Input: part model. Units: mm. Frame: model coordinates. Face numbers are marked on the shaded views. A direction names the side the tool comes from. Give positions to 0.01 mm unless a question says otherwise; leave off trailing zeros. Loops run counter-clockwise (first coordinate to the right, second up) from the corner with the lowest first, then second, coordinate; pieces in that order, holes last. Notation, with made-up numbers: (74.5, 19.25) -> (95.5, 19.25) arc R15 cw to (95.5, 32.25) -> close; hole circle Ø1 at (63.25, 64). An arc over 180 degrees is marked (long way). Answer in a Markdown table with one row per item. Add a question column.
```python
from build123d import *

# Parameters (mm, degrees)
BOSS_EXTRUDE1_DEPTH       = 20
SHELL1_T                  = -3.3
SHELL1_THICKNESS_2_FACE_W = 33.4
SHELL1_THICKNESS_2_FACE_H = 36.7
SHELL1_THICKNESS_2_DEPTH  = 6.7
SHELL1_THICKNESS_3_FACE_W = 36.7
SHELL1_THICKNESS_3_FACE_H = 33.4
SHELL1_THICKNESS_3_DEPTH  = 3.1
CUT_EXTRUDE1_REACH        = 84.439
SKETCH2_R                 = 6.65
CUT_EXTRUDE2_REACH        = 74.967
SKETCH3_R                 = 6.65
FILLET1_R                 = 2


with BuildPart() as part:
    # Sketch1 → Boss-Extrude1 (new, symmetric)
    with BuildSketch(Plane.XY):
        Polygon((0, -24), (0, 0), (16.970562748, 16.970562748), (-11.313708499, 45.254833996), (-40, 16.568542495), (-40, -24), align=None)
    extrude(amount=BOSS_EXTRUDE1_DEPTH, both=True)

    # Shell1
    shell1_openings = [part.faces().sort_by_distance(p)[0] for p in [
        (-40, -3.715728753, 0),
        (-25.656854249, 30.911688245, 0),
    ]]
    offset(amount=SHELL1_T, openings=shell1_openings, kind=Kind.INTERSECTION)

    # Shell1 thickness 2 face (on inner face of the shell) → Shell1 thickness 2 (add)
    with BuildSketch(Plane(origin=(-21.65, -20.7, 0), x_dir=(0, 0, -1), z_dir=(0, -1, 0))):
        Rectangle(SHELL1_THICKNESS_2_FACE_W, SHELL1_THICKNESS_2_FACE_H)
    extrude(amount=-SHELL1_THICKNESS_2_DEPTH)

    # Shell1 thickness 3 face (on inner face of the shell) → Shell1 thickness 3 (add)
    with BuildSketch(Plane(origin=(-0.671751442, 29.945972183, 0), x_dir=(-0.707106781187, 0.707106781187, 0), z_dir=(0.707106781187, 0.707106781187, 0))):
        Rectangle(SHELL1_THICKNESS_3_FACE_W, SHELL1_THICKNESS_3_FACE_H)
    extrude(amount=-SHELL1_THICKNESS_3_DEPTH)

    # Sketch2 → Cut-Extrude1 (cut, up to next)
    with BuildSketch(Plane.XZ.offset(24), mode=Mode.PRIVATE) as cut_extrude1_sk1:
        with Locations(Location((-20, 0, 0), (0, 0, 270))):
            Circle(SKETCH2_R)
    cut_extrude1_tool1 = extrude(cut_extrude1_sk1.sketch, amount=-CUT_EXTRUDE1_REACH, mode=Mode.PRIVATE) & part.part
    add(cut_extrude1_tool1.solids().sort_by_distance((-20, -24, 0))[0], mode=Mode.SUBTRACT)

    # Sketch3 → Cut-Extrude2 (cut, up to next)
    with BuildSketch(Plane(origin=(16.970562748, 16.970562748, 0), x_dir=(0, 0, -1), z_dir=(0.7071067811865488, 0.7071067811865462, 0)), mode=Mode.PRIVATE) as cut_extrude2_sk1:
        with Locations(Location((0, 20, 0), (0, 0, 90))):
            Circle(SKETCH3_R)
    cut_extrude2_tool1 = extrude(cut_extrude2_sk1.sketch, amount=-CUT_EXTRUDE2_REACH, mode=Mode.PRIVATE) & part.part
    add(cut_extrude2_tool1.solids().sort_by_distance((2.828427, 31.112698, 0))[0], mode=Mode.SUBTRACT)

    # Fillet1
    fillet1_edges = [part.edges().sort_by_distance(p)[0] for p in [
        (0, 0, 0),
        (8.485281374, 8.485281374, 20),
        (-25.656854249, 30.911688245, 20),
        (-3.3, 1.366904756, 0),
        (-40, -3.715728753, 20),
        (-40, -3.715728753, -20),
        (-25.656854249, 30.911688245, -20),
        (8.485281374, 8.485281374, -20),
        (0, -12, -20),
        (0, -12, 20),
    ]]
    fillet(fillet1_edges, radius=FILLET1_R)


solid = part.part
```
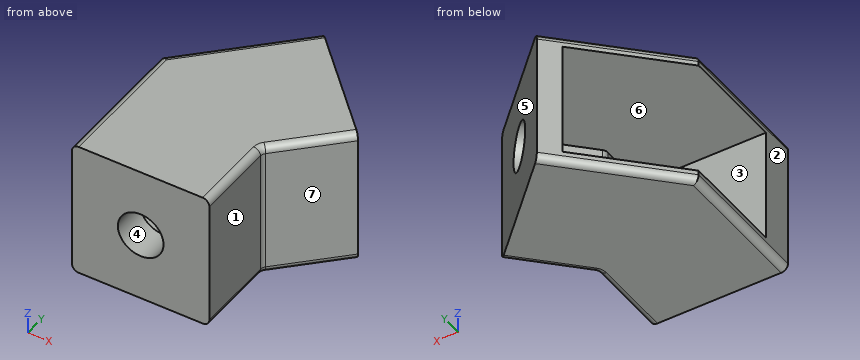
1) Reachability of the marked faces 1, 2 and 3 from +Z, -Z, +X, -X, +Y, -Y: full face, straight path, thin tool, end or side. Return the list, or none.
2) Section D-D on z = -2.5. Output: boundary loops of the cut face in (x, y), and give its area (3 significant figures).
3) Pin query (flat end, axial travel): pin 1 (3 mm diameter, centred on y = 4, z = -6.5, fed in from -X); pin 2 (4.5 mm diameter, centred on y = -3.5, z = -1.5, fed in from -X); pin 3 (1 mm diameter, centred on x = -17.5, z = -3.5, fed in from -Y); pin 4 (1 mm diameter, centred on y = 18.5, z = 12, fed in from -X). Return the tip coordinate at first contact, or that it passes through.
4) Pull-direction query (Y, two-part tool) for the marked faces 4, 5, 6 and 7; classes: +Y half, -Y half, draft (parallel to the pull), parting line (faces both ways), or undercut.
5) Section A-A on z = 3. Output: boundary loops of the cut face in (x, y) (3 decimals).
6) Section B-B on y = -13. Output: boundary loops of the cut face in (x, z), and give its area (3 significant figures).
7) Material intervals for line 1 along X through (y, z) = (-20, 0); line 2 along Z through (x, y) = (-22.5, 30); line 3 along X through (y, z) = (-8.5, 8), sorted ascending.
8) Section C-C on z = 8. Output: boundary loops of the cut face in (x, y).
Working result:
| question | item | result |
|---|---|---|
| 1 | face 1 | +Z, -Z, +X, -Y |
| 1 | face 2 | +Z, -Z, -X, +Y, -Y |
| 1 | face 3 | -X |
| 2 | outline | (-40, -24) -> (-26.16, -24) -> (-26.16, -14) -> (-40, -14) -> close; (-15.84, 40.73) -> (-6.05, 30.94) -> (-1.53, 35.47) -> (-11.31, 45.25) -> close; (-13.84, -24) -> (0, -24) -> (0, -0.83) arc R2 cw to (0.59, 0.59) -> (16.97, 16.97) -> (7.19, 26.76) -> (2.66, 22.23) -> (10.11, 14.78) -> (-2.71, 1.95) arc R2 ccw to (-3.3, 0.54) -> (-3.3, -14) -> (-13.84, -14) -> close |
| 2 | area | 563 mm2 |
| 3 | pin 1 | stops at x = -2.17 |
| 3 | pin 2 | stops at x = -3.3 |
| 3 | pin 3 | passes through |
| 3 | pin 4 | stops at x = 5.89 |
| 4 | face 4 | draft |
| 4 | face 5 | +Y half |
| 4 | face 6 | undercut |
| 4 | face 7 | -Y half |
| 5 | outline | (-40, -24) -> (-25.935, -24) -> (-25.935, -14) -> (-40, -14) -> close; (-15.839, 40.729) -> (-5.894, 30.784) -> (-1.368, 35.309) -> (-11.314, 45.255) -> close; (-14.065, -24) -> (0, -24) -> (0, -0.828) arc R2 cw to (0.586, 0.586) -> (16.971, 16.971) -> (7.025, 26.916) -> (2.5, 22.391) -> (10.112, 14.779) -> (-2.714, 1.953) arc R2 ccw to (-3.3, 0.538) -> (-3.3, -14) -> (-14.065, -14) -> close |
| 6 | outline | (-40, -18) arc R2 ccw to (-38, -20) -> (-2, -20) arc R2 ccw to (0, -18) -> (0, 18) arc R2 ccw to (-2, 20) -> (-38, 20) arc R2 ccw to (-40, 18) -> (-40, 16.7) -> (-3.3, 16.7) -> (-3.3, -16.7) -> (-40, -16.7) -> close |
| 6 | area | 371 mm2 |
| 7 | line 1 | x = -40 to -26.65, -13.35 to 0 |
| 7 | line 2 | z = -20 to -16.7, 16.7 to 20 |
| 7 | line 3 | x = -3.3 to 0 |
| 8 | outline | (-40, -24) -> (0, -24) -> (0, -0.83) arc R2 cw to (0.59, 0.59) -> (16.97, 16.97) -> (-11.31, 45.25) -> (-15.84, 40.73) -> (10.11, 14.78) -> (-2.71, 1.95) arc R2 ccw to (-3.3, 0.54) -> (-3.3, -14) -> (-40, -14) -> close |
